```python
from build123d import *

# Parameters (mm, degrees)
EXTRUDE_1_DEPTH = 100


with BuildPart() as part:
    # 草图1 → 凸台-拉伸1 (new body)
    with BuildSketch(Plane.XY):
        with BuildLine():
            Line((-18.780003001, 7.154207574), (-18.780003001, 5.354207574))
            ThreePointArc((-18.780003001, 5.354207574), (-18.926449611, 5.000654183), (-19.280003001, 4.854207574))
            Line((-19.280003001, 4.854207574), (-19.680003001, 4.854207574))
            ThreePointArc((-19.680003001, 4.854207574), (-20.033556392, 5.000654183), (-20.180003001, 5.354207574))
            Line((-20.180003001, 5.354207574), (-20.180003001, 18.954207574))
            ThreePointArc((-20.180003001, 18.954207574), (-19.740663173, 20.014867745), (-18.680003001, 20.454207574))
            Line((-18.680003001, 20.454207574), (-5.080003001, 20.454207574))
            ThreePointArc((-5.080003001, 20.454207574), (-4.726449611, 20.307760964), (-4.580003001, 19.954207574))
            Line((-4.580003001, 19.954207574), (-4.580003001, 19.554207574))
            ThreePointArc((-4.580003001, 19.554207574), (-4.726449611, 19.200654183), (-5.080003001, 19.054207574))
            Line((-5.080003001, 19.054207574), (-6.880003001, 19.054207574))
            Line((-6.880003001, 19.054207574), (-6.880003001, 8.704207574))
            ThreePointArc((-6.880003001, 8.704207574), (-6.367439869, 7.466770707), (-5.130003001, 6.954207574))
            Line((-5.130003001, 6.954207574), (4.769996999, 6.954207574))
            ThreePointArc((4.769996999, 6.954207574), (6.007433866, 7.466770707), (6.519996999, 8.704207574))
            Line((6.519996999, 8.704207574), (6.519996999, 19.054207574))
            Line((6.519996999, 19.054207574), (4.719996999, 19.054207574))
            ThreePointArc((4.719996999, 19.054207574), (4.366443608, 19.200654183), (4.219996999, 19.554207574))
            Line((4.219996999, 19.554207574), (4.219996999, 19.954207574))
            ThreePointArc((4.219996999, 19.954207574), (4.366443608, 20.307760964), (4.719996999, 20.454207574))
            Line((4.719996999, 20.454207574), (18.319996999, 20.454207574))
            ThreePointArc((18.319996999, 20.454207574), (19.38065717, 20.014867745), (19.819996999, 18.954207574))
            Line((19.819996999, 18.954207574), (19.819996999, 5.354207574))
            ThreePointArc((19.819996999, 5.354207574), (19.673550389, 5.000654183), (19.319996999, 4.854207574))
            Line((19.319996999, 4.854207574), (18.919996999, 4.854207574))
            ThreePointArc((18.919996999, 4.854207574), (18.566443608, 5.000654183), (18.419996999, 5.354207574))
            Line((18.419996999, 5.354207574), (18.419996999, 7.154207574))
            Line((18.419996999, 7.154207574), (8.069996999, 7.154207574))
            ThreePointArc((8.069996999, 7.154207574), (6.832560131, 6.641644441), (6.319996999, 5.404207574))
            Line((6.319996999, 5.404207574), (6.319996999, -4.495792426))
            ThreePointArc((6.319996999, -4.495792426), (6.832560131, -5.733229293), (8.069996999, -6.245792426))
            Line((8.069996999, -6.245792426), (18.419996999, -6.245792426))
            Line((18.419996999, -6.245792426), (18.419996999, -4.445792426))
            ThreePointArc((18.419996999, -4.445792426), (18.566443608, -4.092239036), (18.919996999, -3.945792426))
            Line((18.919996999, -3.945792426), (19.319996999, -3.945792426))
            ThreePointArc((19.319996999, -3.945792426), (19.673550389, -4.092239036), (19.819996999, -4.445792426))
            Line((19.819996999, -4.445792426), (19.819996999, -18.045792426))
            ThreePointArc((19.819996999, -18.045792426), (19.38065717, -19.106452598), (18.319996999, -19.545792426))
            Line((18.319996999, -19.545792426), (4.719996999, -19.545792426))
            ThreePointArc((4.719996999, -19.545792426), (4.366443608, -19.399345817), (4.219996999, -19.045792426))
            Line((4.219996999, -19.045792426), (4.219996999, -18.645792426))
            ThreePointArc((4.219996999, -18.645792426), (4.366443608, -18.292239036), (4.719996999, -18.145792426))
            Line((4.719996999, -18.145792426), (6.519996999, -18.145792426))
            Line((6.519996999, -18.145792426), (6.519996999, -7.795792426))
            ThreePointArc((6.519996999, -7.795792426), (6.007433866, -6.558355559), (4.769996999, -6.045792426))
            Line((4.769996999, -6.045792426), (-5.130003001, -6.045792426))
            ThreePointArc((-5.130003001, -6.045792426), (-6.367439869, -6.558355559), (-6.880003001, -7.795792426))
            Line((-6.880003001, -7.795792426), (-6.880003001, -18.145792426))
            Line((-6.880003001, -18.145792426), (-5.080003001, -18.145792426))
            ThreePointArc((-5.080003001, -18.145792426), (-4.726449611, -18.292239036), (-4.580003001, -18.645792426))
            Line((-4.580003001, -18.645792426), (-4.580003001, -19.045792426))
            ThreePointArc((-4.580003001, -19.045792426), (-4.726449611, -19.399345817), (-5.080003001, -19.545792426))
            Line((-5.080003001, -19.545792426), (-18.680003001, -19.545792426))
            ThreePointArc((-18.680003001, -19.545792426), (-19.740663173, -19.106452598), (-20.180003001, -18.045792426))
            Line((-20.180003001, -18.045792426), (-20.180003001, -4.445792426))
            ThreePointArc((-20.180003001, -4.445792426), (-20.033556392, -4.092239036), (-19.680003001, -3.945792426))
            Line((-19.680003001, -3.945792426), (-19.280003001, -3.945792426))
            ThreePointArc((-19.280003001, -3.945792426), (-18.926449611, -4.092239036), (-18.780003001, -4.445792426))
            Line((-18.780003001, -4.445792426), (-18.780003001, -6.245792426))
            Line((-18.780003001, -6.245792426), (-8.430003001, -6.245792426))
            ThreePointArc((-8.430003001, -6.245792426), (-7.192566134, -5.733229293), (-6.680003001, -4.495792426))
            Line((-6.680003001, -4.495792426), (-6.680003001, 5.404207574))
            ThreePointArc((-6.680003001, 5.404207574), (-7.192566134, 6.641644441), (-8.430003001, 7.154207574))
            Line((-8.430003001, 7.154207574), (-18.780003001, 7.154207574))
        make_face()
        with BuildLine():
            Line((-8.280003001, 19.054207574), (-17.780003001, 19.054207574))
            ThreePointArc((-17.780003001, 19.054207574), (-18.487109783, 18.761314355), (-18.780003001, 18.054207574))
            Line((-18.780003001, 18.054207574), (-18.780003001, 8.554207574))
            Line((-18.780003001, 8.554207574), (-8.280003001, 8.554207574))
            Line((-8.280003001, 8.554207574), (-8.280003001, 19.054207574))
        make_face(mode=Mode.SUBTRACT)
        with BuildLine():
            Line((-4.581369224, 3.58278159), (-5.443828842, 4.445241208))
            ThreePointArc((-5.443828842, 4.445241208), (-5.48330386, 5.757508433), (-4.171036636, 5.718033415))
            Line((-4.171036636, 5.718033415), (-3.308577018, 4.855573796))
            ThreePointArc((-3.308577018, 4.855573796), (-0.180003001, 5.854207574), (2.948571015, 4.855573796))
            Line((2.948571015, 4.855573796), (3.887675086, 5.794677867))
            ThreePointArc((3.887675086, 5.794677867), (5.160467292, 5.718033415), (5.083822839, 4.445241208))
            Line((5.083822839, 4.445241208), (4.221363221, 3.58278159))
            ThreePointArc((4.221363221, 3.58278159), (5.219996999, 0.454207574), (4.221363221, -2.674366443))
            Line((4.221363221, -2.674366443), (5.083822839, -3.536826061))
            ThreePointArc((5.083822839, -3.536826061), (5.123297857, -4.849093285), (3.811030633, -4.809618267))
            Line((3.811030633, -4.809618267), (2.948571015, -3.947158649))
            ThreePointArc((2.948571015, -3.947158649), (-0.180003001, -4.945792426), (-3.308577018, -3.947158649))
            Line((-3.308577018, -3.947158649), (-4.171036636, -4.809618267))
            ThreePointArc((-4.171036636, -4.809618267), (-5.48330386, -4.849093285), (-5.443828842, -3.536826061))
            Line((-5.443828842, -3.536826061), (-4.581369224, -2.674366443))
            ThreePointArc((-4.581369224, -2.674366443), (-5.580003001, 0.454207574), (-4.581369224, 3.58278159))
        make_face(mode=Mode.SUBTRACT)
        with BuildLine():
            Line((7.919996999, 19.054207574), (17.419996999, 19.054207574))
            ThreePointArc((17.419996999, 19.054207574), (18.12710378, 18.761314355), (18.419996999, 18.054207574))
            Line((18.419996999, 18.054207574), (18.419996999, 8.554207574))
            Line((18.419996999, 8.554207574), (7.919996999, 8.554207574))
            Line((7.919996999, 8.554207574), (7.919996999, 19.054207574))
        make_face(mode=Mode.SUBTRACT)
        with BuildLine():
            Line((-8.280003001, -18.145792426), (-17.780003001, -18.145792426))
            ThreePointArc((-17.780003001, -18.145792426), (-18.487109783, -17.852899208), (-18.780003001, -17.145792426))
            Line((-18.780003001, -17.145792426), (-18.780003001, -7.645792426))
            Line((-18.780003001, -7.645792426), (-8.280003001, -7.645792426))
            Line((-8.280003001, -7.645792426), (-8.280003001, -18.145792426))
        make_face(mode=Mode.SUBTRACT)
        with BuildLine():
            Line((7.919996999, -18.145792426), (17.419996999, -18.145792426))
            ThreePointArc((17.419996999, -18.145792426), (18.12710378, -17.852899208), (18.419996999, -17.145792426))
            Line((18.419996999, -17.145792426), (18.419996999, -7.645792426))
            Line((18.419996999, -7.645792426), (7.919996999, -7.645792426))
            Line((7.919996999, -7.645792426), (7.919996999, -18.145792426))
        make_face(mode=Mode.SUBTRACT)
    extrude(amount=EXTRUDE_1_DEPTH)


solid = part.part
```
For this review, take the finished solid that the model builds, in its own axes (mm). Coordinates: 2 decimals unless noted, no trailing zeros. Write each loop counter-clockwise with the first axis right and the second up, starting at its lowest first coordinate (ties: lowest second). Pieces come first, ordered by that corner, then holes. Notation, with made-up numbers: (49, 86.25) - (70, 86.25) arc R12 ccw to (70, 94.25) - close; hole circle Ø4 at (11, 39.25). An arc over 180 degrees is marked (long way). Answer in a Markdown table with one row per item. Add a question column.
Q1. We need section B-B, the plane x = 9.5. State the section outline as (y, z) points.
Q2. Draft analysis for pull direction X (two halves, no side actions). For faces 1 (the flat face through (11, 20.454, 49)), 2 (the flat face through (-20.18, 12, 49)), 3 (the flat face through (18.42, 6, 49)), state which applies: +X half, -X half, draft (parallel to the pull), parting line (faces both ways), or undercut.
Q3. We need section D-D, the plane z = 54.5. Count the separate pieces of the cut face and the enclosed holes in it, and give its area (3 significant figures).
Q4. For P1, Ø3, axis at y = 2.5, z = 39, coming from the +X side; P2, Ø5, axis at y = -1, z = 56, coming from the -X side; P3, Ø1, axis at x = 1.5, z = 32, coming from the -Y side, all flat-tipped, find the tip position at first contact; note any pin that passes through.
Q5. We need section A-A, the plane y = -11.5. State the section outline as (x, z) points.
Q6. For probe 1 along X at (y, z) = (-14, 92.5); probe 2 along Y at (x, z) = (-11.5, 79.5); probe 3 along Y at (x, z) = (18.5, 54), list the stretches that pass through material, from the lowest coordinate up.
Q7. We need section C-C, the plane y = 1.5. State the section outline as (x, z) points, and give its area (3 significant figures).
Answer list:
| question | item | result |
|---|---|---|
| 1 | outline | (-19.55, 0) - (-18.15, 0) - (-18.15, 100) - (-19.55, 100) - close; (-7.65, 0) - (-6.25, 0) - (-6.25, 100) - (-7.65, 100) - close; (7.15, 0) - (8.55, 0) - (8.55, 100) - (7.15, 100) - close; (19.05, 0) - (20.45, 0) - (20.45, 100) - (19.05, 100) - close |
| 2 | face 1 | draft |
| 2 | face 2 | -X half |
| 2 | face 3 | undercut |
| 3 | separate pieces | 1 |
| 3 | enclosed holes | 5 |
| 3 | area | 359 mm2 |
| 4 | P1 | stops at x = 6.32 |
| 4 | P2 | stops at x = -6.68 |
| 4 | P3 | stops at y = -6.05 |
| 5 | outline | (-20.18, 0) - (-18.78, 0) - (-18.78, 100) - (-20.18, 100) - close; (-8.28, 0) - (-6.88, 0) - (-6.88, 100) - (-8.28, 100) - close; (6.52, 0) - (7.92, 0) - (7.92, 100) - (6.52, 100) - close; (18.42, 0) - (19.82, 0) - (19.82, 100) - (18.42, 100) - close |
| 6 | probe 1 | x = -20.18 to -18.78, -8.28 to -6.88, 6.52 to 7.92, 18.42 to 19.82 |
| 6 | probe 2 | y = -19.55 to -18.15, -7.65 to -6.25, 7.15 to 8.55, 19.05 to 20.45 |
| 6 | probe 3 | y = -19.53 to -4.17, 5.08 to 20.44 |
| 7 | outline | (-6.68, 0) - (-5.48, 0) - (-5.48, 100) - (-6.68, 100) - close; (5.12, 0) - (6.32, 0) - (6.32, 100) - (5.12, 100) - close |
| 7 | area | 240 mm2 |
